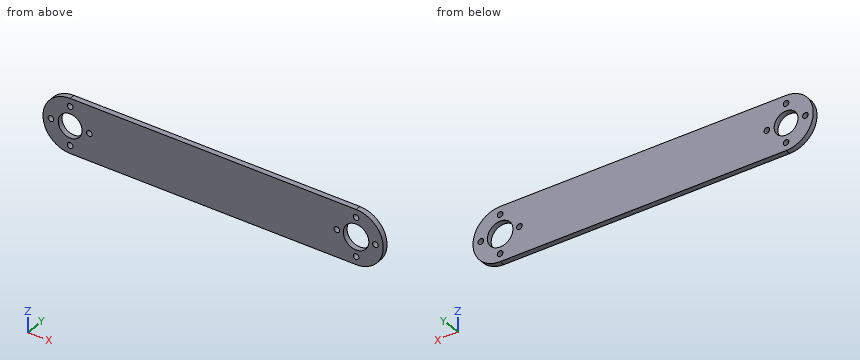
```python
from build123d import *

# Parameters (mm, degrees)
SKETCH1_R           = 7
SKETCH1_R_2         = 7.5
BOSS_EXTRUDE1_DEPTH = 3.175
SKETCH2_R           = 1.65
CUT_EXTRUDE1_DEPTH  = 10


with BuildPart() as part:
    # Sketch1 → Boss-Extrude1 (new body)
    with BuildSketch(Plane(origin=(0, 0, 0), x_dir=(1, 0, 0), z_dir=(0, 1, 0))):
        with BuildLine():
            Line((0, 0), (168, 0))
            ThreePointArc((168, 0), (184, 16), (168, 32))
            Line((168, 32), (0, 32))
            ThreePointArc((0, 32), (-16, 16), (0, 0))
        make_face()
        with Locations(Location((0, 16, 0), (0, 0, 270))):
            Circle(SKETCH1_R, mode=Mode.SUBTRACT)
        with Locations(Location((168, 16, 0), (0, 0, 270))):
            Circle(SKETCH1_R_2, mode=Mode.SUBTRACT)
    extrude(amount=BOSS_EXTRUDE1_DEPTH)

    # Sketch2 → Cut-Extrude1 (cut)
    with BuildSketch(Plane(origin=(0, 3.175, 0), x_dir=(1, 0, 0), z_dir=(0, 1, 0))):
        with Locations(Location((156.686291501, 16, 0), (0, 0, 270))):
            Circle(SKETCH2_R)
        with Locations(Location((168, 27.313708499, 0), (0, 0, 270))):
            Circle(SKETCH2_R)
        with Locations(Location((-11.313708499, 16, 0), (0, 0, 270))):
            Circle(SKETCH2_R)
        with Locations(Location((0, 27.313708499, 0), (0, 0, 270))):
            Circle(SKETCH2_R)
        with Locations(Location((11.313708499, 16, 0), (0, 0, 270))):
            Circle(SKETCH2_R)
        with Locations(Location((0, 4.686291501, 0), (0, 0, 270))):
            Circle(SKETCH2_R)
        with Locations(Location((168, 4.686291501, 0), (0, 0, 270))):
            Circle(SKETCH2_R)
        with Locations(Location((179.313708499, 16, 0), (0, 0, 270))):
            Circle(SKETCH2_R)
    extrude(amount=-CUT_EXTRUDE1_DEPTH, mode=Mode.SUBTRACT)


solid = part.part
```
Build history of the part. All positions in model axes, mm. Round coordinates to 2 decimals unless told otherwise and drop trailing zeros. Loops run counter-clockwise (first coordinate to the right, second up) from the corner with the lowest first, then second, coordinate; pieces in that order, holes last.
Item 1: Drill centre lines: line 1 along X through (y, z) = (2.8, -18.5); line 2 along X through (y, z) = (1.9, -5); line 3 along Z through (x, y) = (10, 2.75). Where is each one in solid material? Low to high.
Item 2: Saw through at A-A (z = -16). List the corners of the cut face in (x, y) (3 decimals), then the cut area to 3 significant figures.
Item 3: Saw through at B-B (y = 2.6). State how many separate pieces and enclosed holes the cut face has, then the cut area to 3 significant figures.
Item 4: Pin check, flat tip, straight feed: P1, Ø1.5, axis at y = 3, z = -8.5, coming from the +X side. Stop position of the tip, or through.
Worked answers:
1. line 1: x = -15.8 to -6.54, 6.54 to 160.93, 175.07 to 183.8
1. line 2: x = -11.62 to -1.62, 1.62 to 166.38, 169.62 to 179.62
1. line 3: z = -32 to -17, -15 to 0
2. outline: (-16, 0) - (-12.964, 0) - (-12.964, 3.175) - (-16, 3.175) - close; (-9.664, 0) - (-7, 0) - (-7, 3.175) - (-9.664, 3.175) - close; (7, 0) - (9.664, 0) - (9.664, 3.175) - (7, 3.175) - close; (12.964, 0) - (155.036, 0) - (155.036, 3.175) - (12.964, 3.175) - close; (158.336, 0) - (160.5, 0) - (160.5, 3.175) - (158.336, 3.175) - close; (175.5, 0) - (177.664, 0) - (177.664, 3.175) - (175.5, 3.175) - close; (180.964, 0) - (184, 0) - (184, 3.175) - (180.964, 3.175) - close
2. area: 501 mm2
3. separate pieces: 1
3. enclosed holes: 10
3. area: 5,780 mm2
4. P1: stops at x = 182.51
